```python
from build123d import *

# Parameters (mm, degrees)
SKETCH1_R           = 1.5
BOSS_EXTRUDE1_DEPTH = 3
SKETCH2_W           = 1.5
SKETCH2_H           = 15.964561632
BOSS_EXTRUDE2_DEPTH = 5


with BuildPart() as part:
    # Sketch1 → Boss-Extrude1 (new body)
    with BuildSketch(Plane(origin=(0, 0, 0), x_dir=(1, 0, 0), z_dir=(0, 1, 0))):
        Polygon((-8.266979, 7.982280816), (-8.266979, -7.982280816), (-3.266979, -7.982280816), (8.266979, -7.982280816), (8.266979, -6.599979816), (8.266979, 6.600020184), (8.266979, 7.982280816), (-3.266979, 7.982280816), align=None)
        with Locations(Location((-5.766979, 4.682321184, 0), (0, 0, 270))):
            Circle(SKETCH1_R, mode=Mode.SUBTRACT)
        with Locations(Location((-5.766979, -4.682280816, 0), (0, 0, 270))):
            Circle(SKETCH1_R, mode=Mode.SUBTRACT)
        Polygon((-2.766979, -6.649979816), (-2.766979, 6.600020184), (6.266979, 6.650020184), (6.266979, -6.599979816), align=None, mode=Mode.SUBTRACT)
    extrude(amount=BOSS_EXTRUDE1_DEPTH)

    # Sketch2 → Boss-Extrude2 (add)
    with BuildSketch(Plane(origin=(0, 0, 0), x_dir=(1, 0, 0), z_dir=(0, 1, 0))):
        with Locations((9.016979, 0)):
            Rectangle(SKETCH2_W, SKETCH2_H)
    extrude(amount=BOSS_EXTRUDE2_DEPTH)


solid = part.part
```
Check sheet for the modelled part. Datum: model origin and axes. Units: mm. A direction names the side the tool comes from. Coordinates: 2 decimals unless noted, no trailing zeros. Order: outer loops, then holes, each group sorted by start corner. A loop starts at its lowest first (then second) coordinate and runs counter-clockwise, first axis right, second up. Notation, with made-up numbers: M 65,-5.75 L 85,-5.75 A24 cw 85,5.25 Z; hole C 59,78 d8. An arc over 180 degrees is marked long. Write each question's results on one line, items separated by ' | '. Start each with the question number.
1. Cross-section at D-D on x = -0.75. Record the cut outline in (y, z), and give its area (3 significant figures).
2. Mould release check, pull along Z, two halves, no side actions. Record for faces 1 (the face through (-4.28, 1.48, 4.49)), 2 (the face through (1, 1, -7.982)), 3 (the face through (1, 1, 7.982)), 4 (the face through (-3, 0, 0)): +Z half, -Z half, draft (parallel to the pull), parting line (faces both ways), or undercut.
3. Cross-section at C-C on z = 2. Record the cut outline in (x, y).
4. Material ranges on probe 1 along X at (y, z) = (0.5, 2); probe 2 along X at (y, z) = (2.35, -5.75); probe 3 along X at (y, z) = (1.85, 4), recorded low to high.
5. Cross-section at A-A on z = -3.5. Record the cut outline in (x, y), and give its area (3 significant figures).
6. Go/stop test with flat-tipped pins: P1, Ø1, axis at y = 4, z = -1.5, coming from the -X side; P2, Ø2, axis at x = 8, z = 2, coming from the -Y side; P3, Ø2.5, axis at x = -5.77, z = 4.68, coming from the -Y side. Record where each tip stops, or that it passes through.
7. Access from +Z, -Z, +X, -X, +Y, -Y to the whole of each face (thin tool, end or side, straight path). Record for faces 5 (the face through (8.267, 4, 0)), 6 (the face through (9.767, 2, 0)), 7 (the face through (-2.767, 1, 0)).
8. Cross-section at B-B on x = -5.5. Record the cut outline in (y, z).
Checks:
1) outline: M 0,-7.98 L 3,-7.98 L 3,-6.61 L 0,-6.61 Z; M 0,6.64 L 3,6.64 L 3,7.98 L 0,7.98 Z | area: 8.14 mm²
2) face 1: undercut | face 2: -Z half | face 3: +Z half | face 4: draft
3) outline: M -8.27,0 L -2.77,0 L -2.77,3 L -8.27,3 Z; M 6.27,0 L 9.77,0 L 9.77,5 L 8.27,5 L 8.27,3 L 6.27,3 Z
4) probe 1: x = -8.27 to -2.77, 6.27 to 9.77 | probe 2: x = -8.27 to -6.82, -4.71 to -2.77, 6.27 to 9.77 | probe 3: x = -8.27 to -7.1, -4.43 to -2.77, 6.27 to 9.77
5) outline: M -8.27,0 L -6.69,0 L -6.69,3 L -8.27,3 Z; M -4.84,0 L -2.77,0 L -2.77,3 L -4.84,3 Z; M 6.27,0 L 9.77,0 L 9.77,5 L 8.27,5 L 8.27,3 L 6.27,3 Z | area: 24.5 mm²
6) P1: stops at x = 8.27 | P2: stops at y = 0 | P3: passes through
7) face 5: +Z, -Z, -X, +Y | face 6: +Z, -Z, +X, +Y, -Y | face 7: +Y, -Y
8) outline: M 0,-7.98 L 3,-7.98 L 3,-6.16 L 0,-6.16 Z; M 0,-3.21 L 3,-3.21 L 3,3.21 L 0,3.21 Z; M 0,6.16 L 3,6.16 L 3,7.98 L 0,7.98 Z
